Model file for the job. Use its own axes, mm. A direction names the side the tool comes from. Coordinates: 2 decimals unless noted, no trailing zeros. Loops run counter-clockwise (first coordinate to the right, second up) from the corner with the lowest first, then second, coordinate; pieces in that order, holes last.
from build123d import *

# Parameters (mm, degrees)
F2_SIZE2 = 0.25
F2_SIZE  = 0.25


with BuildPart() as f1:
    # F0 (on Front) → F1 (revolve)
    with BuildSketch(Plane.XZ):
        Polygon((12.3, -2), (-12.3, -2), (-12.3, -3), (-10.3, -3), (-10.3, -4), (10.3, -4), (10.3, -3), (12.3, -3), align=None)
    revolve(axis=Axis((-53.131774, 0, 0), (1, 0, 0)))

    # F2
    f2_edges = [f1.edges().sort_by_distance(p)[0] for p in [
        (12.3, 0, 2),
        (-12.3, 0, 2),
        (0, 0, -2),
    ]]
    chamfer(f2_edges, length=F2_SIZE, length2=F2_SIZE2)


solid = f1.part
Q1. Slice it at A-A (y = 0). List the corners of the cut face in (x, z), and give its area (3 significant figures).
Answers:
outline: (-12.3, -3) - (-10.3, -3) - (-10.3, -4) - (10.3, -4) - (10.3, -3) - (12.3, -3) - (12.3, -2.25) - (12.05, -2) - (-12.05, -2) - (-12.3, -2.25) - close; (-12.3, 2.25) - (-12.05, 2) - (12.05, 2) - (12.3, 2.25) - (12.3, 3) - (10.3, 3) - (10.3, 4) - (-10.3, 4) - (-10.3, 3) - (-12.3, 3) - close
area: 90.3 mm2
Q2. Which spindle directions (+Z, -Z, +X, -X, +Y, -Y) get a long thin tool onto all of the face, cutting with end or side? Do faces 1 (the flat face through (-10.3, 3, 1)), 2 (the cylindrical face through (11, 0, 3)), 3 (the cylindrical face through (0.144, -3.905, 0.867)). Say none if no direction does.
Answers:
face 1: -X
face 2: +X
face 3: +X, -X
Q3. Slice it at D-D (z = 2.5). List the corners of the cut face in (x, y), and give its area (3 significant figures).
Answers:
outline: (-12.3, -1.66) - (-10.3, -1.66) - (-10.3, -3.12) - (10.3, -3.12) - (10.3, -1.66) - (12.3, -1.66) - (12.3, 1.66) - (10.3, 1.66) - (10.3, 3.12) - (-10.3, 3.12) - (-10.3, 1.66) - (-12.3, 1.66) - close
area: 142 mm2
Q4. Flat gauge pins, fed straight in: P1, Ø4, axis at x = -1.5, z = -2.5, coming from the +Y side; P2, Ø2.5, axis at y = -1, z = -1, coming from the -X side; P3, Ø1.5, axis at x = -9, z = -2.5, coming from the +Y side. Where does each tip first touch, or does it go through?
Answers:
P1: stops at y = 3.97
P2: stops at x = -12.3
P3: stops at y = 3.6
Q5. Mould opens along Y. For faces 4 (the flat face through (10.3, 3, -1)), 5 (the cylindrical face through (-11, 0, 3)), 6 (the cylindrical face through (0, -2, 0)) say: +Y half, -Y half, draft (parallel to the pull), parting line (faces both ways), or undercut.
Answers:
face 4: draft
face 5: parting line
face 6: undercut
Q6. Drill centre lines: line 1 (Y direction, x = -1.25, z = 0); line 2 (Z direction, x = 5, y = 1.5); line 3 (Y direction, x = 11, z = 0.75). Where is each one in solid material? Low to high.
Answers:
line 1: y = -4 to -2, 2 to 4
line 2: z = -3.71 to -1.32, 1.32 to 3.71
line 3: y = -2.9 to -1.85, 1.85 to 2.9
Q7. Slice it at C-C (x = -9). List the corners of the cut face in (y, z).
Answers:
outline: circle Ø8 at (0, 0); hole circle Ø4 at (0, 0)
